```python
from build123d import *

# Parameters (mm, degrees)
CROQUIS1_W              = 19
CROQUIS1_H              = 15
SALIENTE_EXTRUIR1_DEPTH = 7
CROQUIS3_W              = 19
CROQUIS3_H              = 3.8
CORTAR_EXTRUIR1_DEPTH   = 37.9
CROQUIS4_R              = 1
CORTAR_EXTRUIR2_DEPTH   = 51.9


with BuildPart() as part:
    # Croquis1 → Saliente-Extruir1 (new body)
    with BuildSketch(Plane(origin=(0, 0, 0), x_dir=(1, 0, 0), z_dir=(0, 1, 0))):
        Polygon((16.592354246, -24.663454956), (16.592354246, 24.436543518), (8.592354246, 24.436543518), (8.592354246, 14.886544281), (-10.407645754, 14.886544281), (-10.407645754, 24.436543518), (-18.407645754, 24.436543518), (-18.407645754, -24.663454956), (-10.407645754, -24.663454956), (-10.407645754, -15.113455719), (8.592354246, -15.113455719), (8.592354246, -24.663454956), align=None)
        with Locations((-0.907645754, -0.113455719)):
            Rectangle(CROQUIS1_W, CROQUIS1_H, mode=Mode.SUBTRACT)
    extrude(amount=SALIENTE_EXTRUIR1_DEPTH)

    # Croquis3 → Cortar-Extruir1 (cut)
    with BuildSketch(Plane.XY.offset(15.113455719)):
        with Locations((-0.907645754, 5.1)):
            Rectangle(CROQUIS3_W, CROQUIS3_H)
    extrude(amount=-CORTAR_EXTRUIR1_DEPTH, mode=Mode.SUBTRACT)

    # Croquis4 → Cortar-Extruir2 (cut)
    with BuildSketch(Plane.XY.offset(24.663454956)):
        with Locations((12.592354246, 3.5)):
            Circle(CROQUIS4_R)
        with Locations((-14.407645754, 3.5)):
            Circle(CROQUIS4_R)
    extrude(amount=-CORTAR_EXTRUIR2_DEPTH, mode=Mode.SUBTRACT)


solid = part.part
```
Model file for the job. Use its own axes, mm. A direction names the side the tool comes from. Coordinates: 2 decimals unless noted, no trailing zeros. Order: outer loops, then holes, each group sorted by start corner. A loop starts at its lowest first (then second) coordinate and runs counter-clockwise, first axis right, second up. Notation, with made-up numbers: (14.5, 2.5) - (67.5, 2.5) arc R19 cw to (67.5, 10.5) - close; hole circle Ø6 at (2, -29.5). An arc over 180 degrees is marked (long way). Return JSON: item names as keys, results as strings. Group by question number.
1) Saw through at A-A, the plane z = -16.5. Write the cut outline in (x, y).
2) Saw through at D-D, the plane z = 12. Write the cut outline in (x, y), plus the area to 3 significant figures.
3) Tool access for faces 1 (the flat face through (8.592, 3, 0)), 2 (the flat face through (-1, 3.2, 11)), 3 (the flat face through (-1, 2, 7.613)), 4 (the flat face through (-1, 2, -14.887)): list every direction of +Z, -Z, +X, -X, +Y, -Y with a clear straight run to the whole face (end or side of a thin tool).
4) Flat gauge pins, fed straight in: P1, Ø3, axis at x = -1.5, y = 1, coming from the +Z side; P2, Ø1.6, axis at x = -3.5, y = 1, coming from the -Z side; P3, Ø6, axis at x = 1.5, z = -12, coming from the +Y side. Where does each tip first touch, or does it go through?
5) Saw through at C-C, the plane y = 1.25. Write the cut outline in (x, z), plus the area to 3 significant figures.
6) Probe line 1 (X direction, y = 5, z = 7); line 2 (Y direction, x = 12.5, z = 19); line 3 (Z direction, x = -8.5, y = 1.75). List the from-to ranges inside material, lowest first. Write a range as from..to.
7) Mould opens along Y. For faces 5 (the cylindrical face through (13.546, 3.8, 0.457)), 6 (the cylindrical face through (-13.454, 3.8, 0.457)), 7 (the flat face through (-1, 2, 15.113)), 8 (the flat face through (-1, 0, -11)) say: released by +Y, released by -Y, zero draft, split by the parting line, or undercut.
8) Saw through at B-B, the plane x = -8. Write the cut outline in (y, z).
Values found:
{
 "1": {"outline": "(-18.41, 0) - (-10.41, 0) - (-10.41, 7) - (-18.41, 7) - close; (8.59, 0) - (16.59, 0) - (16.59, 7) - (8.59, 7) - close; hole circle Ø2 at (-14.41, 3.5); hole circle Ø2 at (12.59, 3.5)"},
 "2": {"outline": "(-18.41, 0) - (16.59, 0) - (16.59, 7) - (8.59, 7) - (8.59, 3.2) - (-10.41, 3.2) - (-10.41, 7) - (-18.41, 7) - close; hole circle Ø2 at (-14.41, 3.5); hole circle Ø2 at (12.59, 3.5)", "area": "167 mm²"},
 "3": {"face 1": "+Y", "face 2": "+Z, -Z, +Y", "face 3": "+Y, -Y", "face 4": "-Z, +Y, -Y"},
 "4": {"P1": "stops at z = 15.11", "P2": "stops at z = -14.89", "P3": "stops at y = 3.2"},
 "5": {"outline": "(-18.41, -24.44) - (-10.41, -24.44) - (-10.41, -14.89) - (8.59, -14.89) - (8.59, -24.44) - (16.59, -24.44) - (16.59, 24.66) - (8.59, 24.66) - (8.59, 15.11) - (-10.41, 15.11) - (-10.41, 24.66) - (-18.41, 24.66) - close; hole (-10.41, -7.39) - (8.59, -7.39) - (8.59, 7.61) - (-10.41, 7.61) - close", "area": "1,070 mm²"},
 "6": {"line 1": "x = -18.41..-10.41, 8.59..16.59", "line 2": "y = 0..2.5, 4.5..7", "line 3": "z = -14.89..-7.39, 7.61..15.11"},
 "7": {"face 5": "undercut", "face 6": "undercut", "face 7": "zero draft", "face 8": "released by -Y"},
 "8": {"outline": "(0, -14.89) - (3.2, -14.89) - (3.2, -7.39) - (0, -7.39) - close; (0, 7.61) - (3.2, 7.61) - (3.2, 15.11) - (0, 15.11) - close"}
}
